from build123d import *

# Parameters (mm, degrees)
BASPROSKE_W        = 4
BASPROSKE_H        = 14.4
TOOTHCUT_DEPTH     = 21.753794834
TEETHCUTS_COUNT    = 30
TEETHCUTS_ANGLE    = 348
BORE_DEPTH         = 50.0000508
CUT_EXTRUDE2_START = -10
CUT_EXTRUDE2_DEPTH = 10
CUT_EXTRUDE3_START = -2.47
SKETCH3_R          = 1.5
CUT_EXTRUDE3_DEPTH = 2.47


with BuildPart() as part:
    # BasProSke → Base-Revolve (revolve)
    with BuildSketch(Plane(origin=(0, 0, 0), x_dir=(1, 0, 0), z_dir=(0, 1, 0)), mode=Mode.PRIVATE) as base_revolve_sk:
        with Locations((2, 7.2)):
            Rectangle(BASPROSKE_W, BASPROSKE_H)
    revolve(base_revolve_sk.sketch.rotate(Axis((-10, 0, 0), (1, 0, 0)), 180), axis=Axis((-10, 0, 0), (1, 0, 0)))

    # TooCutSke → ToothCut (cut, through all)
    with BuildSketch(Plane(origin=(0, 0, 0), x_dir=(0, 0, -1), z_dir=(1, 0, 0))):
        with BuildLine():
            ThreePointArc((0.502005058, 12.363812799), (0, 12.374), (-0.502005058, 12.363812799))
            ThreePointArc((-0.502005058, 12.363812799), (-0.740487606, 13.404090158), (-1.178907792, 14.377146503))
            ThreePointArc((-1.178907792, 14.377146503), (0, 14.4254), (1.178907792, 14.377146503))
            ThreePointArc((1.178907792, 14.377146503), (0.740487606, 13.404090158), (0.502005058, 12.363812799))
        make_face()
    toothcut = extrude(amount=TOOTHCUT_DEPTH, mode=Mode.SUBTRACT)

    # TeethCuts: ToothCut ×30 about axis
    teethcuts_axis = Axis((-10, 0, 0), (1, 0, 0))
    for i in range(1, TEETHCUTS_COUNT):
        add(toothcut.rotate(teethcuts_axis, i * TEETHCUTS_ANGLE / (TEETHCUTS_COUNT - 1)), mode=Mode.SUBTRACT)

    # BorSke → Bore (cut, symmetric)
    with BuildSketch(Plane(origin=(0, 0, 0), x_dir=(0, 0, -1), z_dir=(1, 0, 0))):
        with BuildLine():
            Line((-1.160818677, -0.95), (1.160818677, -0.95))
            ThreePointArc((1.160818677, -0.95), (0, 1.5), (-1.160818677, -0.95))
        make_face()
    extrude(amount=BORE_DEPTH, both=True, mode=Mode.SUBTRACT)

    # Sketch1 → Cut-Extrude2 (cut)
    with BuildSketch(Plane(origin=(4, 0, 0), x_dir=(0, 0, -1), z_dir=(1, 0, 0)).offset(CUT_EXTRUDE2_START)):
        with BuildLine():
            Line((-9.19567407, 8.279822123), (-11.837430087, 9.990379384))
            ThreePointArc((-11.837430087, 9.990379384), (-15.480248321, -0.542534064), (-11.108982601, -10.79457905))
            Line((-11.108982601, -10.79457905), (-9.083189008, -8.403068097))
            ThreePointArc((-9.083189008, -8.403068097), (-12.373718737, -0.083430299), (-9.19567407, 8.279822123))
        make_face()
        with BuildLine():
            Line((9.083189008, -8.403068097), (11.108982601, -10.79457905))
            ThreePointArc((11.108982601, -10.79457905), (15.480248321, -0.542534064), (11.837430087, 9.990379384))
            Line((11.837430087, 9.990379384), (9.19567407, 8.279822123))
            ThreePointArc((9.19567407, 8.279822123), (12.373718737, -0.083430299), (9.083189008, -8.403068097))
        make_face()
    extrude(amount=CUT_EXTRUDE2_DEPTH, mode=Mode.SUBTRACT)

    # Sketch3 → Cut-Extrude3 (cut)
    with BuildSketch(Plane.ZY.offset(CUT_EXTRUDE3_START)):
        with Locations(Location((0, 0, 0), (0, 0, 320.703519761))):
            Circle(SKETCH3_R)
    extrude(amount=CUT_EXTRUDE3_DEPTH, mode=Mode.SUBTRACT)


solid = part.part
Geometry check sheet. Reference: the model listing, model coordinates, mm. A direction names the side the tool comes from. Give positions to 0.01 mm unless a question says otherwise; leave off trailing zeros. Loops run counter-clockwise (first coordinate to the right, second up) from the corner with the lowest first, then second, coordinate; pieces in that order, holes last. Notation, with made-up numbers: M 16.25,36.5 L 50.25,36.5 A8 cw 50.25,42.5 Z; hole C 89,29.5 d10. An arc over 180 degrees is marked long. Answer as a JSON object with one key per item and string values. Group by question number.
Item 1: Sectioned sample at D-D on z = 6. Record the boundary of the cut face in (x, y), plus the area to 3 significant figures.
Item 2: Sectioned sample at C-C on z = 8.5. Record the boundary of the cut face in (x, y).
Item 3: Sectioned sample at A-A on z = 0. Record the boundary of the cut face in (x, y), plus the area to 3 significant figures.
Item 4: Gauge pin test, flat ends, axial feed: pin 1 (1 mm diameter, centred on x = 2, y = -2, fed in from +Z); pin 2 (2 mm diameter, centred on x = 1.5, z = 0, fed in from +Y); pin 3 (1.7 mm diameter, centred on x = 3.5, z = 0, fed in from +Y). Record the tip position at first contact, or that the pin passes through.
Item 5: Sectioned sample at B-B on y = 0. Record the boundary of the cut face in (x, z), plus the area to 3 significant figures.
Item 6: Material ranges on L1, parallel to Z at x = 1.4, y = 0; L2, parallel to Y at x = 1.1, z = -9.5; L3, parallel to Z at x = 0.65, y = 12.75, recorded low to high.
Item 7: Mould release check, pull along Z, two halves, no side actions. Record for faces 4 (the cylindrical face through (1.972, -13.237, 2.066)), 5 (the flat face through (0, 0, -3)): pulls with the +Z half, pulls with the -Z half, needs draft (parallel to the pull), parting line crosses it, or undercut.
Item 8: Access from +Z, -Z, +X, -X, +Y, -Y to the whole of each face (thin tool, end or side, straight path). Record for faces 1 (the cylindrical face through (1.97, 13.4, -0.74)), 2 (the cylindrical face through (1.972, -11.307, -5.027)), 3 (the cylindrical face through (1.97, -13.4, 0.74)).
Findings below:
{
 "1": {"outline": "M 0,-11.8 L 4,-11.8 L 4,11.8 L 0,11.8 Z", "area": "94.4 mm2"},
 "2": {"outline": "M 0,-10.42 L 4,-10.42 L 4,10.42 L 0,10.42 Z"},
 "3": {"outline": "M 0,-12.37 L 4,-12.37 L 4,-0.95 L 2.47,-0.95 L 2.47,-1.5 L 0,-1.5 Z; M 0,1.5 L 4,1.5 L 4,12.37 L 0,12.37 Z", "area": "87.8 mm2"},
 "4": {"pin 1": "z = 12.28", "pin 2": "y = 14.04", "pin 3": "y = 13.7"},
 "5": {"outline": "M 0,-12.37 L 4,-12.37 L 4,-1.5 L 0,-1.5 Z; M 0,1.5 L 4,1.5 L 4,12.37 L 0,12.37 Z", "area": "87.0 mm2"},
 "6": {"L1": "-12.37 to -1.5, 1.5 to 12.37", "L2": "-10.82 to -9.58, -7.93 to 7.93, 9.58 to 10.82", "L3": "-4.79 to -3.39, -2.1 to -0.57, 0.57 to 2.1, 3.39 to 4.79"},
 "7": {"face 4": "undercut", "face 5": "needs draft"},
 "8": {"face 1": "+X, -X, +Y", "face 2": "+X, -X", "face 3": "+X, -X, -Y"}
}
